Source: CAD feature listing. Evaluate the final solid. Frame: model axes, mm. A direction names the side the tool comes from. Give positions to 0.01 mm unless a question says otherwise; leave off trailing zeros. Loops run counter-clockwise (first coordinate to the right, second up) from the corner with the lowest first, then second, coordinate; pieces in that order, holes last. Notation, with made-up numbers: M 70.25,72 L 80.25,72 A16 ccw 80.25,91 Z; hole C 65,40 d6. An arc over 180 degrees is marked long. Answer in a Markdown table with one row per item.
```python
from build123d import *

# Parameters (mm, degrees)
F0_W           = 70
F0_H           = 120
F0_R           = 5.5
F1_DEPTH       = 5
F2_D           = 3.1
F2_DEPTH       = 5
F2_CBORE_D     = 6
F2_CBORE_DEPTH = 3
F2_TIP         = 0.9313339595
F3_W           = 13.85
F3_H           = 16.5
F3_R           = 0.5
F4_DEPTH       = 2
F5_DEPTH       = 5
F3_R_2         = 1.55
F6_DEPTH       = 4
F0_W_2         = 76
F0_H_2         = 126
F7_DEPTH       = 60
F8_R           = 5
F9_W           = 11.5
F9_H           = 3
F10_DEPTH      = 3


with BuildPart() as f1:
    # F0 (on Front) → F1 (new body)
    with BuildSketch(Plane.XZ):
        Rectangle(F0_W, F0_H)
        with Locations((0, -16.15)):
            Circle(F0_R, mode=Mode.SUBTRACT)
        with Locations((0, 36.15)):
            Circle(F0_R, mode=Mode.SUBTRACT)
    extrude(amount=-F1_DEPTH)

    # F2
    with Locations(Plane.XZ):
        with Locations((15.5, 51.65), (-15.5, 51.65), (-15.5, 20.65), (15.5, 20.65), (15.5, -0.65), (-15.5, -0.65), (-15.5, -31.65), (15.5, -31.65)):
            CounterBoreHole(F2_D / 2, F2_CBORE_D / 2, F2_CBORE_DEPTH, depth=F2_DEPTH)
            with Locations((0, 0, -(F2_DEPTH + F2_TIP / 2))):  # 118° drill point
                Cone(0, F2_D / 2, F2_TIP, mode=Mode.SUBTRACT)

    # F3 (on face) → F4 (cut)
    with BuildSketch(Plane(origin=(0, 5, 0), x_dir=(-1, 0, 0), z_dir=(0, 1, 0))):
        with BuildLine():
            ThreePointArc((-8.0117101795, 27.9), (-11.5, 36.15), (-8.0117101795, 44.4))
            Line((-8.0117101795, 44.4), (-21.15, 44.4))
            Line((-21.15, 44.4), (-21.15, 27.9))
            Line((-21.15, 27.9), (-8.0117101795, 27.9))
        make_face()
        with Locations((-28.075, 36.15)):
            Rectangle(F3_W, F3_H)
        with BuildLine():
            Line((-5.5, 44.4), (-8.0117101795, 44.4))
            ThreePointArc((-8.0117101795, 44.4), (-11.5, 36.15), (-8.0117101795, 27.9))
            Line((-8.0117101795, 27.9), (-5.5, 27.9))
            Line((-5.5, 27.9), (-5.5, 31.4))
            Line((-5.5, 31.4), (-10, 31.4))
            Line((-10, 31.4), (-10, 40.9))
            Line((-10, 40.9), (-5.5, 40.9))
            Line((-5.5, 40.9), (-5.5, 44.4))
        make_face()
        with Locations((-7.5, 29.9)):
            Circle(F3_R, mode=Mode.SUBTRACT)
        with Locations((-7.5, 42.4)):
            Circle(F3_R, mode=Mode.SUBTRACT)
        with Locations((-28.075, -16.15)):
            Rectangle(F3_W, F3_H)
        with BuildLine():
            Line((-8.0117101795, -7.9), (-21.15, -7.9))
            Line((-21.15, -7.9), (-21.15, -24.4))
            Line((-21.15, -24.4), (-8.0117101795, -24.4))
            ThreePointArc((-8.0117101795, -24.4), (-11.5, -16.15), (-8.0117101795, -7.9))
        make_face()
        with BuildLine():
            Line((-5.5, -7.9), (-8.0117101795, -7.9))
            ThreePointArc((-8.0117101795, -7.9), (-11.5, -16.15), (-8.0117101795, -24.4))
            Line((-8.0117101795, -24.4), (-5.5, -24.4))
            Line((-5.5, -24.4), (-5.5, -20.9))
            Line((-5.5, -20.9), (-10, -20.9))
            Line((-10, -20.9), (-10, -11.4))
            Line((-10, -11.4), (-5.5, -11.4))
            Line((-5.5, -11.4), (-5.5, -7.9))
        make_face()
        with Locations((-7.5, -22.4)):
            Circle(F3_R, mode=Mode.SUBTRACT)
        with Locations((-7.5, -9.9)):
            Circle(F3_R, mode=Mode.SUBTRACT)
    extrude(amount=-F4_DEPTH, mode=Mode.SUBTRACT)

    # F3 (on face) → F5 (cut)
    with BuildSketch(Plane(origin=(0, 5, 0), x_dir=(-1, 0, 0), z_dir=(0, 1, 0))):
        with BuildLine():
            Line((-2.7726341266, 40.9), (-5.5, 40.9))
            Line((-5.5, 40.9), (-10, 40.9))
            Line((-10, 40.9), (-10, 31.4))
            Line((-10, 31.4), (-5.5, 31.4))
            Line((-5.5, 31.4), (-2.7726341266, 31.4))
            ThreePointArc((-2.7726341266, 31.4), (-5.5, 36.15), (-2.7726341266, 40.9))
        make_face()
        with BuildLine():
            Line((-2.7726341266, -11.4), (-5.5, -11.4))
            Line((-5.5, -11.4), (-10, -11.4))
            Line((-10, -11.4), (-10, -20.9))
            Line((-10, -20.9), (-5.5, -20.9))
            Line((-5.5, -20.9), (-2.7726341266, -20.9))
            ThreePointArc((-2.7726341266, -20.9), (-5.5, -16.15), (-2.7726341266, -11.4))
        make_face()
    extrude(amount=-F5_DEPTH, mode=Mode.SUBTRACT)

    # F3 (on face) → F6 (join)
    with BuildSketch(Plane(origin=(0, 5, 0), x_dir=(-1, 0, 0), z_dir=(0, 1, 0))):
        with BuildLine():
            ThreePointArc((-8.0117101795, 44.4), (4.4785786214, 46.7420882517), (11.5, 36.15))
            ThreePointArc((11.5, 36.15), (4.4785786214, 25.5579117483), (-8.0117101795, 27.9))
            Line((-8.0117101795, 27.9), (-21.15, 27.9))
            Line((-21.15, 27.9), (-21.15, 15))
            Line((-21.15, 15), (21.15, 15))
            Line((21.15, 15), (21.15, 57.3))
            Line((21.15, 57.3), (-21.15, 57.3))
            Line((-21.15, 57.3), (-21.15, 44.4))
            Line((-21.15, 44.4), (-8.0117101795, 44.4))
        make_face()
        with Locations((-15.5, 20.65)):
            Circle(F3_R_2, mode=Mode.SUBTRACT)
        with Locations((-15.5, 51.65)):
            Circle(F3_R_2, mode=Mode.SUBTRACT)
        with Locations((15.5, 20.65)):
            Circle(F3_R_2, mode=Mode.SUBTRACT)
        with Locations((15.5, 51.65)):
            Circle(F3_R_2, mode=Mode.SUBTRACT)
        with BuildLine():
            Line((-21.15, 5), (-21.15, -7.9))
            Line((-21.15, -7.9), (-8.0117101795, -7.9))
            ThreePointArc((-8.0117101795, -7.9), (4.4785786214, -5.5579117483), (11.5, -16.15))
            ThreePointArc((11.5, -16.15), (4.4785786214, -26.7420882517), (-8.0117101795, -24.4))
            Line((-8.0117101795, -24.4), (-21.15, -24.4))
            Line((-21.15, -24.4), (-21.15, -37.3))
            Line((-21.15, -37.3), (21.15, -37.3))
            Line((21.15, -37.3), (21.15, 5))
            Line((21.15, 5), (-21.15, 5))
        make_face()
        with Locations((-15.5, -31.65)):
            Circle(F3_R_2, mode=Mode.SUBTRACT)
        with Locations((-15.5, -0.65)):
            Circle(F3_R_2, mode=Mode.SUBTRACT)
        with Locations((15.5, -31.65)):
            Circle(F3_R_2, mode=Mode.SUBTRACT)
        with Locations((15.5, -0.65)):
            Circle(F3_R_2, mode=Mode.SUBTRACT)
    extrude(amount=F6_DEPTH)

    # F0 (on Front) → F7 (join)
    with BuildSketch(Plane.XZ):
        Rectangle(F0_W_2, F0_H_2)
        Rectangle(F0_W, F0_H, mode=Mode.SUBTRACT)
    extrude(amount=-F7_DEPTH)

    # F8
    f8_edges = [f1.edges().sort_by_distance(p)[0] for p in [
        (38, 30, 63),
        (38, 0, 0),
        (0, 0, 63),
        (-38, 30, 63),
        (-38, 0, 0),
    ]]
    fillet(f8_edges, radius=F8_R)

    # F9 (on face) → F10 (join)
    with BuildSketch(Plane(origin=(0, 60, 0), x_dir=(-1, 0, 0), z_dir=(0, 1, 0))):
        with Locations((-27.25, -61.5)):
            Rectangle(F9_W, F9_H)
    extrude(amount=F10_DEPTH)


solid = f1.part
```
Q1. Mould query, pull axis Z, two halves, no side actions, for faces 5 (the cylindrical face through (0, 2, 62)), 6 (the flat face through (33, 61, -62)), 7 (the flat face through (10, 2, 36)). Classes: +Z half, -Z half, draft (parallel to the pull), parting line (faces both ways), or undercut.
Values follow:
| item | result |
|---|---|
| face 5 | +Z half |
| face 6 | draft |
| face 7 | undercut |
Q2. Section query A-A (z = 51.65). Give the number of separate pieces and of enclosed holes in the cut face, plus the area to 3 significant figures.
Values follow:
| item | result |
|---|---|
| separate pieces | 3 |
| enclosed holes | 0 |
| area | 795 mm^2 |
Q3. Section query B-B (y = 50.5). Output: boundary loops of the cut face in (x, z), plus the area to 3 significant figures.
Values follow:
| item | result |
|---|---|
| outline | M -38,-63 L 38,-63 L 38,58 A5 ccw 33,63 L -33,63 A5 ccw -38,58 Z; hole M -35,-60 L 35,-60 L 35,60 L -35,60 Z |
| area | 1,170 mm^2 |
Q4. Section query D-D (x = -9). Output: boundary loops of the cut face in (y, z).
Values follow:
| item | result |
|---|---|
| outline | M 0,-63 L 60,-63 L 60,-60 L 5,-60 L 5,-37.3 L 9,-37.3 L 9,-23.31 L 5,-23.31 L 5,-8.99 L 9,-8.99 L 9,5 L 5,5 L 5,15 L 9,15 L 9,28.99 L 5,28.99 L 5,43.31 L 9,43.31 L 9,57.3 L 5,57.3 L 5,60 L 60,60 L 60,63 L 5,63 A5 ccw 0,58 Z |
Q5. Section query C-C (z = -52.5). Output: boundary loops of the cut face in (x, y).
Values follow:
| item | result |
|---|---|
| outline | M -38,5 A5 ccw -33,0 L 33,0 A5 ccw 38,5 L 38,60 L 35,60 L 35,5 L -35,5 L -35,60 L -38,60 Z |
Q6. Reachability of faces 1 (the flat face through (0, 32, 63)), 2 (the flat face through (6, 2, -11.4)), 3 (the flat face through (0, 7, 57.3)), 4 (the cylindrical face through (-17.881, 1.479, 18.825)) from +Z, -Z, +X, -X, +Y, -Y: full face, straight path, thin tool, end or side. Return the list, or none.
Values follow:
| item | result |
|---|---|
| face 1 | +Z, +X, -X, +Y, -Y |
| face 2 | +Y, -Y |
| face 3 | +Y |
| face 4 | -Y |
Q7. Contact query for flat-ended pins moving along their axis: pin 1 Ø8 at (x, z) = (20, -13.5) entering from +Y; pin 2 Ø5 at (x, z) = (-15.5, 20.65) entering from -Y; pin 3 Ø3 at (x, z) = (-15.5, 20.65) entering from -Y; pin 4 Ø6 at (x, z) = (-4, -21) entering from +Y. Output: stop coordinate, or through.
Values follow:
| item | result |
|---|---|
| pin 1 | y = 3 |
| pin 2 | y = 3 |
| pin 3 | through |
| pin 4 | y = 5 |
Q8. Ray query, probe 1 along X at (y, z) = (6.75, 51.65); probe 2 along Z at (x, y) = (17, 37); probe 3 along Z at (x, y) = (-15.5, 1.15). Return the intervals inside material, ascending. Write a range as from..to.
Values follow:
| item | result |
|---|---|
| probe 1 | -38..-35, -21.15..-17.05, -13.95..13.95, 17.05..21.15, 35..38 |
| probe 2 | -63..-60, 60..63 |
| probe 3 | -63..-34.65, -28.65..-3.65, 2.35..17.65, 23.65..48.65, 54.65..61.19 |
